Build history of the part. All positions in model axes, mm. Face numbers are marked on the shaded views. A direction names the side the tool comes from. Round coordinates to 2 decimals unless told otherwise and drop trailing zeros. Write each loop counter-clockwise with the first axis right and the second up, starting at its lowest first coordinate (ties: lowest second). Pieces come first, ordered by that corner, then holes. Notation, with made-up numbers: (-15, 57) -> (24, 57) arc R23 cw to (24, 95) -> close; hole circle Ø4 at (-33.5, 76.5). An arc over 180 degrees is marked (long way). Answer in a Markdown table with one row per item.
```python
from build123d import *

# Parameters (mm, degrees)
SKETCH1_W           = 56
SKETCH1_H           = 36.73970361
SKETCH1_W_2         = 50
SKETCH1_H_2         = 30.73970361
BOSS_EXTRUDE1_DEPTH = 25.4
SKETCH2_W           = 56
SKETCH2_H           = 36.73970361
BOSS_EXTRUDE2_DEPTH = 4
FILLET1_R           = 10
SKETCH3_W           = 56
SKETCH3_H           = 3
CUT_EXTRUDE1_DEPTH  = 28


with BuildPart() as part:
    # Sketch1 → Boss-Extrude1 (new body)
    with BuildSketch(Plane.XY):
        with Locations((0, -51.412888934)):
            Rectangle(SKETCH1_W, SKETCH1_H)
        with Locations((0, -51.412888934)):
            Rectangle(SKETCH1_W_2, SKETCH1_H_2, mode=Mode.SUBTRACT)
    extrude(amount=BOSS_EXTRUDE1_DEPTH)

    # Sketch2 → Boss-Extrude2 (add)
    with BuildSketch(Plane.XY.offset(25.4)):
        with Locations((0, -51.412888934)):
            Rectangle(SKETCH2_W, SKETCH2_H)
    extrude(amount=-BOSS_EXTRUDE2_DEPTH)

    # Fillet1
    fillet1_edges = [part.edges().sort_by_distance(p)[0] for p in [
        (28, -51.412888934, 25.4),
        (-28, -51.412888934, 25.4),
        (0, -69.782740739, 25.4),
    ]]
    fillet(fillet1_edges, radius=FILLET1_R)

    # Sketch3 → Cut-Extrude1 (cut)
    with BuildSketch(Plane(origin=(0, 0, 0), x_dir=(-1, 0, 0), z_dir=(0, 0, -1))):
        with Locations((0, -34.543037129)):
            Rectangle(SKETCH3_W, SKETCH3_H)
    extrude(amount=-CUT_EXTRUDE1_DEPTH, mode=Mode.SUBTRACT)


solid = part.part
```
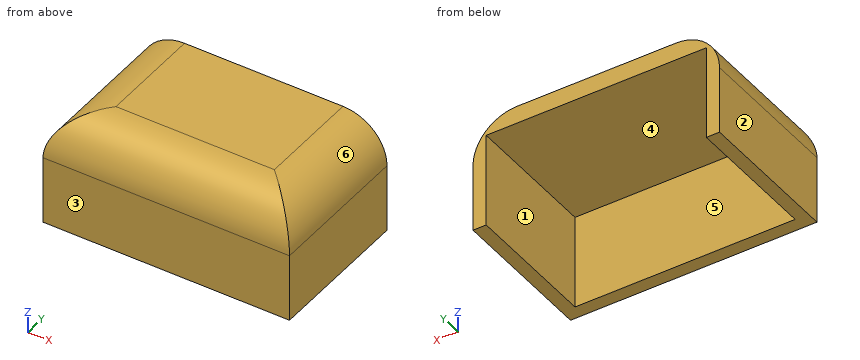
Q1. Two-plate mould, pull along X, no slides. Class the marked faces 1, 2, 3 and 4: released by +X, released by -X, zero draft, split by the parting line, or undercut.
A:
| item | result |
|---|---|
| face 1 | undercut |
| face 2 | released by -X |
| face 3 | zero draft |
| face 4 | undercut |
Q2. Saw through at C-C on z = 8.5. Write the cut outline in (x, y).
A:
| item | result |
|---|---|
| outline | (-28, -69.78) -> (28, -69.78) -> (28, -36.04) -> (25, -36.04) -> (25, -66.78) -> (-25, -66.78) -> (-25, -36.04) -> (-28, -36.04) -> close |
Q3. Saw through at D-D on y = -62.5. Write the cut outline in (x, z), plus the area to 3 significant figures.
A:
| item | result |
|---|---|
| outline | (-28, 0) -> (-25, 0) -> (-25, 21.4) -> (25, 21.4) -> (25, 0) -> (28, 0) -> (28, 15.4) arc R10 ccw to (20.72, 25.02) -> (-20.72, 25.02) arc R10 ccw to (-28, 15.4) -> close |
| area | 295 mm² |
Q4. Which spindle directions (+Z, -Z, +X, -X, +Y, -Y) get a long thin tool onto all of the face, cutting with end or side? Do the marked faces 5 and 6. Say none if no direction does.
A:
| item | result |
|---|---|
| face 5 | -Z, +Y |
| face 6 | +Z, +X, +Y, -Y |
Q5. Saw through at A-A on x = -14. Write the cut outline in (y, z), plus the area to 3 significant figures.
A:
| item | result |
|---|---|
| outline | (-69.78, 0) -> (-66.78, 0) -> (-66.78, 21.4) -> (-36.04, 21.4) -> (-36.04, 25.4) -> (-59.78, 25.4) arc R10 ccw to (-69.78, 15.4) -> close |
| area | 178 mm² |
Q6. Drop flat-ended pins along their axis: P1, Ø1.5, axis at x = 20, y = -41, coming from the -Z side; P2, Ø2, axis at y = -52, z = 18.5, coming from the -X side; P3, Ø4, axis at x = 22, z = 18, coming from the +Y side. Give the stop position or say it passes through.
A:
| item | result |
|---|---|
| P1 | z = 21.4 |
| P2 | x = -27.78 |
| P3 | y = -66.78 |
Q7. Wall check: line 1 (X direction, y = -39, z = 4); line 2 (Z direction, x = -11.5, y = -60); line 3 (Y direction, x = 22, z = 13.25). Give the ranges that are in metal, low to high. Write a range as [from, to].
A:
| item | result |
|---|---|
| line 1 | [-28, -25], [25, 28] |
| line 2 | [21.4, 25.4] |
| line 3 | [-69.78, -66.78] |
Q8. Saw through at B-B on y = -42.5. Write the cut outline in (x, z).
A:
| item | result |
|---|---|
| outline | (-28, 0) -> (-25, 0) -> (-25, 21.4) -> (25, 21.4) -> (25, 0) -> (28, 0) -> (28, 15.4) arc R10 ccw to (18, 25.4) -> (-18, 25.4) arc R10 ccw to (-28, 15.4) -> close |
